from build123d import *

# Parameters (mm, degrees)
BOSS_EXTRUDE1_DEPTH = 19.05
SKETCH7_R           = 3.3782
CUT_EXTRUDE3_DEPTH  = 233.356054205
BOSS_EXTRUDE3_START = -6.35
BOSS_EXTRUDE3_DEPTH = 19.05
SKETCH11_R          = 3.3782
CUT_EXTRUDE4_DEPTH  = 238.616089602
FILLET4_R           = 3.175


with BuildPart() as part:
    # Sketch1 → Boss-Extrude1 (new body)
    with BuildSketch(Plane.XY):
        with BuildLine():
            Line((-182.9308, 127.79756), (-163.8808, 127.79756))
            Line((-163.8808, 127.79756), (-163.8808, 121.44756))
            Line((-163.8808, 121.44756), (-176.5808, 121.44756))
            Line((-176.5808, 121.44756), (-176.5808, 99.757550505))
            Line((-176.5808, 99.757550505), (-217.8558, 99.757550505))
            Line((-217.8558, 99.757550505), (-217.8558, 121.44756))
            Line((-217.8558, 121.44756), (-230.5558, 121.44756))
            Line((-230.5558, 121.44756), (-230.5558, 127.79756))
            Line((-230.5558, 127.79756), (-211.5058, 127.79756))
            ThreePointArc((-211.5058, 127.79756), (-197.2183, 113.51006), (-182.9308, 127.79756))
        make_face()
    extrude(amount=BOSS_EXTRUDE1_DEPTH)

    # Sketch7 → Cut-Extrude3 (cut, through all)
    with BuildSketch(Plane.XZ.offset(-121.44756)):
        with Locations((-170.2308, 9.525)):
            Circle(SKETCH7_R)
        with Locations((-224.2058, 9.525)):
            Circle(SKETCH7_R)
    extrude(amount=-CUT_EXTRUDE3_DEPTH, mode=Mode.SUBTRACT)

    # Sketch10 → Boss-Extrude3 (add)
    with BuildSketch(Plane(origin=(-163.8808, 0, 0), x_dir=(0, 0, -1), z_dir=(1, 0, 0)).offset(BOSS_EXTRUDE3_START)):
        with BuildLine():
            Line((6.35, 83.882550505), (24.473547486, 83.882550505))
            Line((24.473547486, 83.882550505), (24.473547486, 90.232550505))
            Line((24.473547486, 90.232550505), (11.773547486, 90.232550505))
            ThreePointArc((11.773547486, 90.232550505), (-9.525, 106.107550505), (-30.823547486, 90.232550505))
            Line((-30.823547486, 90.232550505), (-43.523547486, 90.232550505))
            Line((-43.523547486, 90.232550505), (-43.523547486, 83.882550505))
            Line((-43.523547486, 83.882550505), (-25.4, 83.882550505))
            ThreePointArc((-25.4, 83.882550505), (-9.525, 99.757550505), (6.35, 83.882550505))
        make_face()
    boss_extrude3 = extrude(amount=-BOSS_EXTRUDE3_DEPTH)

    # Mirror3: Boss-Extrude3 across plane
    add(boss_extrude3.mirror(Plane(origin=(-197.2183, 0, 0), x_dir=(0, 0, 1), z_dir=(1, 0, 0))))

    # Sketch11 → Cut-Extrude4 (cut, through all)
    with BuildSketch(Plane(origin=(0, 90.232550505, 0), x_dir=(1, 0, 0), z_dir=(0, 1, 0))):
        with Locations(Location((-179.7558, -37.173547486, 0), (0, 0, 270))):
            Circle(SKETCH11_R)
        with Locations(Location((-179.7558, 18.123547486, 0), (0, 0, 270))):
            Circle(SKETCH11_R)
        with Locations(Location((-214.6808, 18.123547486, 0), (0, 0, 270))):
            Circle(SKETCH11_R)
        with Locations(Location((-214.6808, -37.173547486, 0), (0, 0, 270))):
            Circle(SKETCH11_R)
    extrude(amount=-CUT_EXTRUDE4_DEPTH, mode=Mode.SUBTRACT)

    # Fillet4
    fillet4_edges = [part.edges().sort_by_distance(p)[0] for p in [
        (-182.9308, 127.79756, 9.525),
        (-211.5058, 127.79756, 9.525),
        (-189.2808, 101.860282076, 0),
        (-182.9308, 103.963013647, 0),
        (-189.2808, 101.860282076, 19.05),
        (-179.7558, 83.882550505, -6.35),
        (-179.7558, 83.882550505, 25.4),
        (-182.9308, 103.963013647, 19.05),
        (-176.5808, 106.107550505, 9.525),
        (-205.1558, 101.860282076, 0),
        (-211.5058, 103.963013647, 0),
        (-211.5058, 103.963013647, 19.05),
        (-217.8558, 106.107550505, 9.525),
        (-205.1558, 101.860282076, 19.05),
        (-214.6808, 83.882550505, 25.4),
        (-214.6808, 83.882550505, -6.35),
    ]]
    fillet(fillet4_edges, radius=FILLET4_R)


solid = part.part
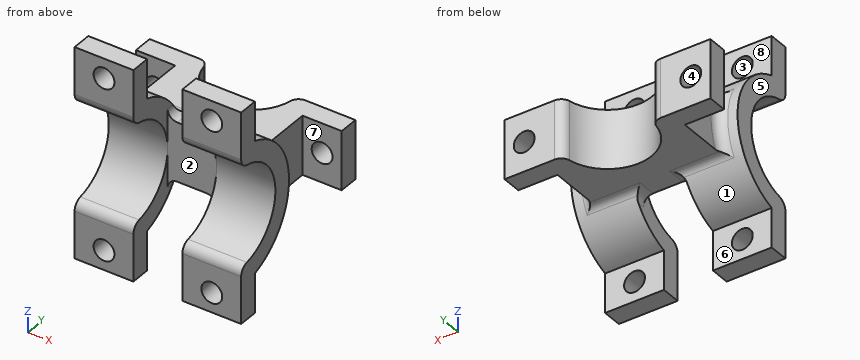
Verification items for the finished model (mm, model axes). Face numbers are marked on the shaded views. A direction names the side the tool comes from. Coordinates: 2 decimals unless noted, no trailing zeros. Write each loop counter-clockwise with the first axis right and the second up, starting at its lowest first coordinate (ties: lowest second). Pieces come first, ordered by that corner, then holes. Notation, with made-up numbers: M 22,32.25 L 26,32.25 A17 ccw 26,65.25 Z; hole C -1,7.5 d9. An arc over 180 degrees is marked long. Use a Markdown table: item, result.
Q1. Set-up check for the marked faces 4, 5, 6, 7 and 8: record each of +Z, -Z, +X, -X, +Y, -Y from which the full face is reachable in a straight line by a thin tool's end or side.
Reply:
| item | result |
|---|---|
| face 4 | +Y |
| face 5 | +Z, -Z, -X, -Y |
| face 6 | -Z, +X, -X, +Y |
| face 7 | +Z, -Z, +X |
| face 8 | +Z, +X, -X, +Y |
Q2. Sectioned sample at B-B, the plane y = 97. Record the boundary of the cut face in (x, z).
Reply:
| item | result |
|---|---|
| outline | M -224.21,-8.42 L -205.16,-8.42 L -205.16,0.58 L -224.21,0.58 Z; M -224.21,18.47 L -205.16,18.47 L -205.16,27.47 L -224.21,27.47 Z; M -189.28,-8.42 L -170.23,-8.42 L -170.23,0.58 L -189.28,0.58 Z; M -189.28,18.47 L -170.23,18.47 L -170.23,27.47 L -189.28,27.47 Z |
Q3. Go/stop test with flat-tipped pins: P1, Ø5.5, axis at y = 96, z = -0.5, coming from the +X side; P2, Ø1.5, axis at x = -204, z = 32, coming from the +Y side; P3, Ø7, axis at y = 115, z = 5.5, coming from the -X side; P4, Ø10, axis at x = -221.5, z = 5.5, coming from the -Y side. Record where each tip stops, or that it passes through.
Reply:
| item | result |
|---|---|
| P1 | stops at x = -170.23 |
| P2 | passes through |
| P3 | stops at x = -217.86 |
| P4 | stops at y = 96.94 |
Q4. Thickness scan on line 1 (Y direction, x = -176, z = -16); line 2 (Z direction, x = -217, y = 114); line 3 (X direction, y = 92.5, z = 26.5). Record the ranges inside material, lowest first.
Reply:
| item | result |
|---|---|
| line 1 | y = 83.88 to 90.23 |
| line 2 | z = 0 to 19.05 |
| line 3 | x = -224.21 to -205.16, -189.28 to -170.23 |
Q5. Sectioned sample at D-D, the plane y = 117.5. Record the boundary of the cut face in (x, z).
Reply:
| item | result |
|---|---|
| outline | M -217.86,0 L -207.12,0 L -207.12,19.05 L -217.86,19.05 Z; M -187.31,0 L -176.58,0 L -176.58,19.05 L -187.31,19.05 Z |
Q6. Draft check along Z on the marked faces 1, 2 and 3. Enter one of: +Z half, -Z half, draft (parallel to the pull), parting line (faces both ways), or undercut.
Reply:
| item | result |
|---|---|
| face 1 | parting line |
| face 2 | draft |
| face 3 | undercut |
Q7. Sectioned sample at A-A, the plane y = 87.5. Record the boundary of the cut face in (x, z).
Reply:
| item | result |
|---|---|
| outline | M -224.21,-24.47 L -205.16,-24.47 L -205.16,-5.93 L -224.21,-5.93 Z; M -224.21,24.98 L -205.16,24.98 L -205.16,43.52 L -224.21,43.52 Z; M -189.28,-24.47 L -170.23,-24.47 L -170.23,-5.93 L -189.28,-5.93 Z; M -189.28,24.98 L -170.23,24.98 L -170.23,43.52 L -189.28,43.52 Z; hole C -214.68,-18.12 d6.76; hole C -214.68,37.17 d6.76; hole C -179.76,-18.12 d6.76; hole C -179.76,37.17 d6.76 |
